Here's how the part is built. I have some questions about the finished solid (model axes, mm). A direction names the side the tool comes from. Coordinates: 2 decimals unless noted, no trailing zeros. Write each loop counter-clockwise with the first axis right and the second up, starting at its lowest first coordinate (ties: lowest second). Pieces come first, ordered by that corner, then holes.
Item 1: I'm going to push flat-ended pins straight in: pin 1 Ø1.2 at (x, y) = (4, -0.5) entering from -Z; pin 2 Ø0.8 at (x, y) = (-2.5, 2) entering from +Z; pin 3 Ø1.2 at (x, y) = (3.5, -1) entering from +Z. Where does each tip first touch, or does it pass through?
Item 2: If I drill on line 1 (Y direction, x = 0, z = 0.65); line 2 (Z direction, x = 1.75, y = 0.95); line 3 (Z direction, x = 4, y = -0.25), over which ranges is the centre line in solid material (lowest first)?
Item 3: If we section it at A-A (x = 0): Please give me the cut outline in (y, z), then the cut area to 3 significant figures.
Item 4: If we section it at B-B (y = 0.6): Please give me the cut outline in (x, z), then the cut area to 3 significant figures.
Item 5: If we section it at C-C (x = 3.98): Please give me the cut outline in (y, z), then the cut area to 4 significant figures.
Item 6: For faces 1 (the face through (4, -1, 0.7)), 2 (the face through (-0.28, -1.27, 0.01)), 3 (the face through (4, -1, -0.7)), which set-ups out of +Z, -Z, +X, -X, +Y, -Y let a thin tool reach every point of the face, with its end or its side?
from build123d import *

# Parameters (mm, degrees)
SKETCH1_R           = 1.3
SKETCH1_R_2         = 0.3
BOSS_EXTRUDE1_DEPTH = 1
SKETCH1_3_R         = 0.7625
BOSS_EXTRUDE2_DEPTH = 0.7
BOSS_EXTRUDE3_DEPTH = 0.6
BOSS_EXTRUDE4_DEPTH = 0.2
SKETCH5_R           = 0.3
BOSS_EXTRUDE5_DEPTH = 0.2


with BuildPart() as part:
    # Sketch1 → Boss-Extrude1 (new body, symmetric)
    with BuildSketch(Plane.XY):
        Circle(SKETCH1_R)
        Circle(SKETCH1_R_2, mode=Mode.SUBTRACT)
    extrude(amount=BOSS_EXTRUDE1_DEPTH, both=True)



with BuildPart() as body_2:
    # Sketch1_3 → Boss-Extrude2 (new body, symmetric)
    with BuildSketch(Plane.XY):
        with Locations((3.98, -0.682)):
            Circle(SKETCH1_3_R)
    extrude(amount=BOSS_EXTRUDE2_DEPTH, both=True)


with BuildPart() as part_1:
    add(part.part)

    add(body_2.part)  # Boss-Extrude3 merges body 2
    # Sketch1_4 → Boss-Extrude3 (add, symmetric)
    with BuildSketch(Plane.XY):
        with BuildLine():
            Line((2.186048651, 0.944502367), (0.219469493, 1.281340369))
            ThreePointArc((0.219469493, 1.281340369), (0.993808417, 0.838060159), (1.3, 0))
            ThreePointArc((1.3, 0), (1.123700283, -0.653680101), (0.642618962, -1.13006233))
            add(Edge.make_bspline(
                [(3.494717907, -1.270139049), (2.819202825, -1.086203937), (1.830443771, -0.782374183), (0.874191176, -0.998376943), (0.642618962, -1.13006233)],
                knots=[0, 0, 0, 0, 0.738093499, 1, 1, 1, 1], degree=3))
            ThreePointArc((3.494717907, -1.270139049), (3.22524382, -0.573605538), (3.679849137, 0.018939162))
            Line((3.679849137, 0.018939162), (2.186048651, 0.944502367))
        make_face()
        with BuildLine():
            ThreePointArc((-1.295848634, -0.103809043), (-1.071749439, 0.735767042), (-0.368782161, 1.24659525))
            Line((-0.368782161, 1.24659525), (-1.915411787, 2.192219906))
            Line((-1.915411787, 2.192219906), (-3.469420101, 2.791170079))
            Line((-3.469420101, 2.791170079), (-3.851452989, 2.234684794))
            Line((-3.851452989, 2.234684794), (-2.734084179, 0.999707022))
            Line((-2.734084179, 0.999707022), (-1.295848634, -0.103809043))
        make_face()
    extrude(amount=BOSS_EXTRUDE3_DEPTH, both=True)



with BuildPart() as body_2_2:
    # Sketch2 → Revolve1 (revolve)
    with BuildSketch(Plane.XY):
        with BuildLine():
            Line((-3.851452989, 2.234684794), (-3.443951242, 2.828269098))
            Line((-3.443951242, 2.828269098), (-3.769598187, 3.051829084))
            Line((-3.769598187, 3.051829084), (-4.833144721, 1.502622153))
            ThreePointArc((-4.833144721, 1.502622153), (-4.424469448, 1.511609143), (-4.303041686, 1.901931501))
            Line((-4.303041686, 1.901931501), (-3.851452989, 2.234684794))
        make_face()
    revolve(axis=Axis((-3.769598187, 3.051829084, 0), (-0.565974648, -0.824422645, 0)))


with BuildPart() as part_2:
    add(part_1.part)

    add(body_2_2.part)  # Revolve2 merges body 2 2
    # Sketch3 → Revolve2 (revolve)
    with BuildSketch(Plane.XY):
        Polygon((-4.2939678, 2.288010094), (-3.684979079, 3.175088861), (-4.437676954, 3.691823714), (-5.046665676, 2.804744948), align=None)
    revolve(axis=Axis((-4.2939678, 2.288010094, 0), (0.565974648, 0.824422645, 0)))

    # Sketch4 → Boss-Extrude4 (add, symmetric)
    with BuildSketch(Plane(origin=(0.30110441, 0.438601438, 0), x_dir=(0.824422645, -0.565974648, 0), z_dir=(0.565974648, 0.824422645, 0))):
        Polygon((-4.185, 0.375277675), (-4.835, 0.75055535), (-5.485, 0.375277675), (-5.485, -0.375277675), (-4.835, -0.75055535), (-4.185, -0.375277675), align=None)
    extrude(amount=BOSS_EXTRUDE4_DEPTH, both=True)

    # Sketch5 → Boss-Extrude5 (add, symmetric)
    with BuildSketch(Plane(origin=(0.41429934, 0.603485967, 0), x_dir=(0.824422645, -0.565974648, 0), z_dir=(0.565974648, 0.824422645, 0))):
        with Locations((-4.835, 0)):
            Circle(SKETCH5_R)
    extrude(amount=BOSS_EXTRUDE5_DEPTH, both=True)


solid = part_2.part
Answer list:
1. pin 1: stops at z = -0.7
1. pin 2: stops at z = 0.6
1. pin 3: stops at z = 0.7
2. line 1: y = -1.3 to -0.3, 0.3 to 1.3
2. line 2: z = -0.6 to 0.6
2. line 3: z = -0.7 to 0.7
3. outline: (-1.3, -1) - (-0.3, -1) - (-0.3, 1) - (-1.3, 1) - close; (0.3, -1) - (1.3, -1) - (1.3, 1) - (0.3, 1) - close
3. area: 4.00 mm2
4. outline: (-2.21, -0.6) - (-1.15, -0.6) - (-1.15, -1) - (1.15, -1) - (1.15, -0.6) - (2.74, -0.6) - (2.74, 0.6) - (1.15, 0.6) - (1.15, 1) - (-1.15, 1) - (-1.15, 0.6) - (-2.21, 0.6) - close
4. area: 7.79 mm2
5. outline: (-1.44, -0.7) - (0.08, -0.7) - (0.08, 0.7) - (-1.44, 0.7) - close
5. area: 2.135 mm2
6. face 1: +Z, +X, +Y, -Y
6. face 2: none
6. face 3: -Z, +X, +Y, -Y
